For this review, use the dimensioned drawing (mm, ordinates from the lowest corner) and the shaded views. Give positions to 0.01 mm unless a question says otherwise; leave off trailing zeros. Loops run counter-clockwise (first coordinate to the right, second up) from the corner with the lowest first, then second, coordinate; pieces in that order, holes last. Notation, with made-up numbers: (-25.5, -26) -> (8.5, -26) arc R8 cw to (8.5, -13) -> close; hole circle Ø6 at (29.5, 79.25). An arc over 180 degrees is marked (long way). Write each question's results on one line, items separated by ' | '. Start each with the question number.
Q1. Insertion check: pin 1 Ø1.5 at (x, z) = (75.5, 4) entering from +Y; pin 2 Ø2 at (y, z) = (76.5, 4) entering from -X; pin 3 Ø2 at (x, z) = (67, 0.5) entering from +Y. Each pin has a flat end and moves straight along its axis. Give the tip position at first contact, or say it passes through.
Q2. We need section A-A (y = 50). Write out the cut boundary in (x, z).
Q3. Wall thickness on L1, parallel to Y at x = 50, z = 2.55; L2, parallel to X at y = 47.5, z = 0.65; L3, parallel to Y at x = 15.5, z = 3.6: over which ranges is each line inside the solid? List them lowest first. Write a range as [from, to].
Q4. We need section C-C (y = 78). Write out the cut boundary in (x, z).
Q5. We need section B-B (x = 50). Write out the cut boundary in (y, z).
Q6. We need section D-D (z = 2.75). Write out the cut boundary in (x, y), plus the area to 3 significant figures.
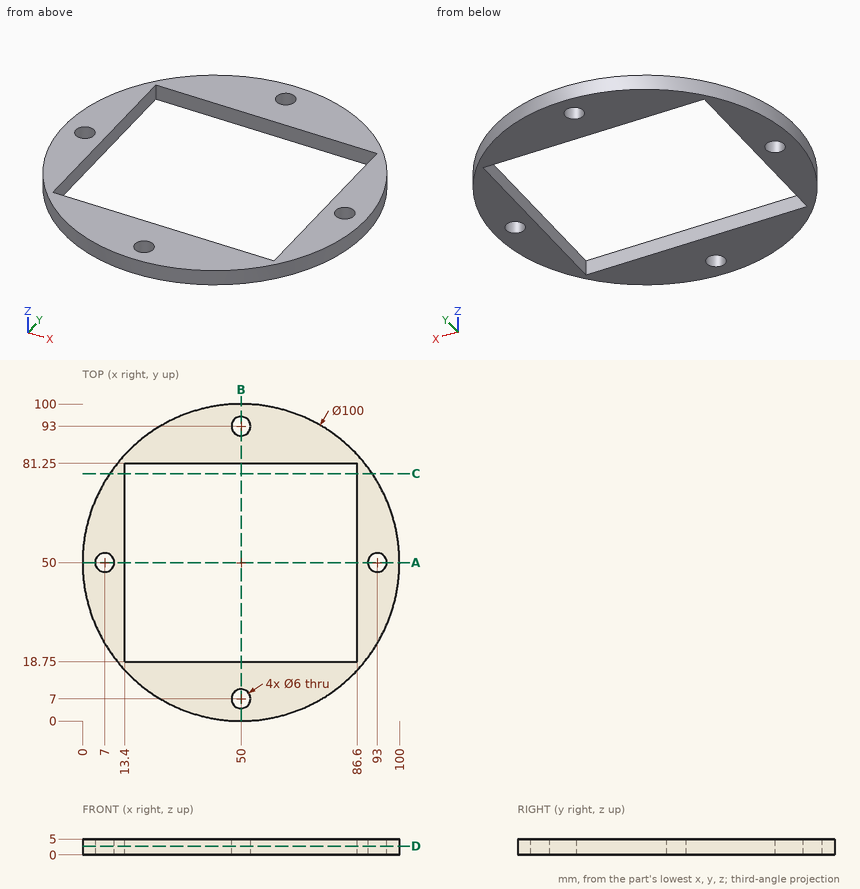
Output:
1) pin 1: y = 93.44 | pin 2: x = 6.99 | pin 3: y = 97.37
2) outline: (0, 0) -> (4, 0) -> (4, 5) -> (0, 5) -> close; (10, 0) -> (13.4, 0) -> (13.4, 5) -> (10, 5) -> close; (86.6, 0) -> (90, 0) -> (90, 5) -> (86.6, 5) -> close; (96, 0) -> (100, 0) -> (100, 5) -> (96, 5) -> close
3) L1: [0, 4], [10, 18.75], [81.25, 90], [96, 100] | L2: [0.06, 5.34], [8.66, 13.4], [86.6, 91.34], [94.66, 99.94] | L3: [13.81, 18.75], [81.25, 86.19]
4) outline: (8.58, 0) -> (13.4, 0) -> (13.4, 5) -> (8.58, 5) -> close; (86.6, 0) -> (91.42, 0) -> (91.42, 5) -> (86.6, 5) -> close
5) outline: (0, 0) -> (4, 0) -> (4, 5) -> (0, 5) -> close; (10, 0) -> (18.75, 0) -> (18.75, 5) -> (10, 5) -> close; (81.25, 0) -> (90, 0) -> (90, 5) -> (81.25, 5) -> close; (96, 0) -> (100, 0) -> (100, 5) -> (96, 5) -> close
6) outline: circle Ø100 at (50, 50); hole circle Ø6 at (7, 50); hole (13.4, 18.75) -> (86.6, 18.75) -> (86.6, 81.25) -> (13.4, 81.25) -> close; hole circle Ø6 at (50, 7); hole circle Ø6 at (50, 93); hole circle Ø6 at (93, 50) | area: 3,170 mm2
